from build123d import *

# Parameters (mm, degrees)
SKETCH_1_W      = 10
SKETCH_1_H      = 3
EXTRUDE_1_DEPTH = 3


with BuildPart() as part:
    # 草图1 → 凸台-拉伸1 (new body)
    with BuildSketch(Plane.XY):
        Polygon((-53, 5), (-53, -5), (-53, -10), (67, -10), (67, -5), (67, 5), (67, 10), (-53, 10), align=None)
        with Locations((-30, 6.5)):
            Rectangle(SKETCH_1_W, SKETCH_1_H, mode=Mode.SUBTRACT)
        with Locations((-45, 6.5)):
            Rectangle(SKETCH_1_W, SKETCH_1_H, mode=Mode.SUBTRACT)
        with Locations((-15, 6.5)):
            Rectangle(SKETCH_1_W, SKETCH_1_H, mode=Mode.SUBTRACT)
        with Locations((0, 6.5)):
            Rectangle(SKETCH_1_W, SKETCH_1_H, mode=Mode.SUBTRACT)
        with Locations((15, 6.5)):
            Rectangle(SKETCH_1_W, SKETCH_1_H, mode=Mode.SUBTRACT)
        with Locations((30, 6.5)):
            Rectangle(SKETCH_1_W, SKETCH_1_H, mode=Mode.SUBTRACT)
        with Locations((45, 6.5)):
            Rectangle(SKETCH_1_W, SKETCH_1_H, mode=Mode.SUBTRACT)
        with Locations((45, -6.5)):
            Rectangle(SKETCH_1_W, SKETCH_1_H, mode=Mode.SUBTRACT)
        with Locations((30, -6.5)):
            Rectangle(SKETCH_1_W, SKETCH_1_H, mode=Mode.SUBTRACT)
        with Locations((15, -6.5)):
            Rectangle(SKETCH_1_W, SKETCH_1_H, mode=Mode.SUBTRACT)
        with Locations((0, -6.5)):
            Rectangle(SKETCH_1_W, SKETCH_1_H, mode=Mode.SUBTRACT)
        with Locations((-15, -6.5)):
            Rectangle(SKETCH_1_W, SKETCH_1_H, mode=Mode.SUBTRACT)
        with Locations((-30, -6.5)):
            Rectangle(SKETCH_1_W, SKETCH_1_H, mode=Mode.SUBTRACT)
        with Locations((-45, -6.5)):
            Rectangle(SKETCH_1_W, SKETCH_1_H, mode=Mode.SUBTRACT)
        with Locations((60, 6.5)):
            Rectangle(SKETCH_1_W, SKETCH_1_H, mode=Mode.SUBTRACT)
        with Locations((60, -6.5)):
            Rectangle(SKETCH_1_W, SKETCH_1_H, mode=Mode.SUBTRACT)
    extrude(amount=EXTRUDE_1_DEPTH)


solid = part.part
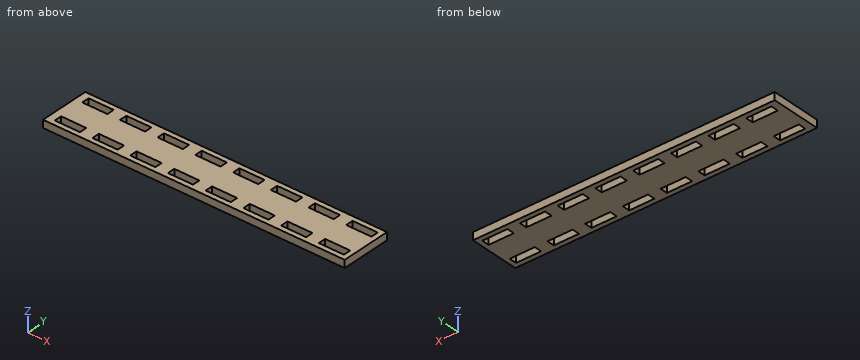
Source: CAD feature listing. Evaluate the final solid. Frame: model axes, mm. Round coordinates to 2 decimals unless told otherwise and drop trailing zeros. Loops run counter-clockwise (first coordinate to the right, second up) from the corner with the lowest first, then second, coordinate; pieces in that order, holes last.
Q1. Ray query, line 1 (Y direction, x = 56, z = 1.1). Return the intervals inside material, ascending.
Q2. Section B-B, the plane z = 2.4. State how many separate pieces and enclosed holes the cut face has, plus the area to 3 significant figures.
Q3. Section A-A, the plane x = 3.5. Return loops of the section in (y, z).
Q4. First-contact query: P1, Ø8, axis at x = 27.5, y = 0, coming from the -Z side. Flat tip, straight axial feed; report the tip coordinate or a pass-through.
Solutions:
1. line 1: y = -10 to -8, -5 to 5, 8 to 10
2. separate pieces: 1
2. enclosed holes: 16
2. area: 1,920 mm2
3. outline: (-10, 0) - (-8, 0) - (-8, 3) - (-10, 3) - close; (-5, 0) - (5, 0) - (5, 3) - (-5, 3) - close; (8, 0) - (10, 0) - (10, 3) - (8, 3) - close
4. P1: stops at z = 0
